from build123d import *

# Parameters (mm, degrees)
F1_DEPTH    = 7
F2_DEPTH    = 8
F3_R        = 3.99999
F4_T1_DEPTH = 20.2030500331
F5_R        = 5
F6_R        = 2.5
F7_DEPTH    = 10
F6_R_2      = 3
F8_DEPTH    = 4.6
F9_R        = 1.7
F10_DEPTH   = 7.001


# Not quite as in the source:
# - a fillet or chamfer that OpenCascade refuses, or shapes differently, is made with other operations: its cross-section is extruded or revolved along the edge and cut away or added
# - a fillet or chamfer is up to 0.001 mm smaller than in the source, because OpenCascade refuses the exact size


with BuildPart() as f1:
    # F0 (on Top) → F1 (new body)
    with BuildSketch(Plane.XY):
        Polygon((-25, -4), (25, -4), (25, 4), (-19.7969499669, 4), (-25, 4), align=None)
    extrude(amount=F1_DEPTH)

    # F0 (on Top) → F2 (join)
    with BuildSketch(Plane.XY):
        Polygon((-15.1648762861, 40.705181399), (-25, 4), (-19.7969499669, 4), (-10.3103645166, 39.4044188907), align=None)
    extrude(amount=F2_DEPTH)

    # F3 (radius 4 in the source; OpenCascade refuses exactly that, so slightly less here)
    f3_edges = [f1.edges().sort_by_distance(p)[0] for p in [
        (25, 4, 3.5),
        (25, -4, 3.5),
        (-25, -4, 3.5),
        (-10.310365, 39.404419, 4),
    ]]
    fillet(f3_edges, radius=F3_R)

    # F4: fillet of radius 5 on 1 edges, made by hand

    # F4_s2 → F4_t1 (cut)
    with BuildSketch(Plane.YZ.offset(-32.5)):
        with BuildLine():
            ThreePointArc((4, 7), (5.4188611699, 7.7434164903), (7, 8))
            Line((7, 8), (4, 8))
            Line((4, 8), (4, 7))
        make_face()
    extrude(amount=F4_T1_DEPTH, mode=Mode.SUBTRACT)

    # F5
    f5_edges = [f1.edges().sort_by_distance(p)[0] for p in [
        (-22.398475, 4, 7),
    ]]
    fillet(f5_edges, radius=F5_R)

    # F6 (on face) → F7 (cut)
    with BuildSketch(Plane(origin=(-24.3253175473, 6.5179491924, 0), x_dir=(-0.2588190451, -0.9659258263, 0), z_dir=(-0.9659258263, 0.2588190451, 0))):
        with Locations((-27.3932271776, 4)):
            Circle(F6_R)
    extrude(amount=-F7_DEPTH, mode=Mode.SUBTRACT)

    # F6 (on face) → F8 (cut)
    with BuildSketch(Plane(origin=(-24.3253175473, 6.5179491924, 0), x_dir=(-0.2588190451, -0.9659258263, 0), z_dir=(-0.9659258263, 0.2588190451, 0))):
        with Locations((-8.3932271776, 4)):
            Circle(F6_R_2)
    extrude(amount=-F8_DEPTH, mode=Mode.SUBTRACT)

    # F9 (on face) → F10 (cut, through all)
    with BuildSketch(Plane.XY.offset(7)):
        with Locations((21, 0)):
            Circle(F9_R)
    extrude(amount=-F10_DEPTH, mode=Mode.SUBTRACT)


solid = f1.part
The listing builds one solid part. Answer for the finished solid, in the listing's coordinates (mm). A direction names the side the tool comes from. Give positions to 0.01 mm unless a question says otherwise; leave off trailing zeros. Loops run counter-clockwise (first coordinate to the right, second up) from the corner with the lowest first, then second, coordinate; pieces in that order, holes last. Notation, with made-up numbers: (-34.75, 32) - (-15.75, 32) arc R21 ccw to (-15.75, 59) - close; hole circle Ø2 at (-11, 43.25). An arc over 180 degrees is marked (long way). Use one line per item in the form item = value.
1. Which of the six approach directions +Z, -Z, +X, -X, +Y, -Y give full straight-line access (tool end or side, diameter ignored) to faces 1 (the face through (-17.699, 13.475, 4.042)), 2 (the face through (0, -4, 3)), 3 (the face through (1, 4, 3))?
Calculated:
face_1 = none
face_2 = +Z, -Z, +X, -X, -Y
face_3 = +Z, -Z, +X
2. Find the intervals of material crossed by line 1 along Y through (x, z) = (21, 5.25); line 2 along Z through (x, y) = (-4, 1); line 3 along Y through (x, z) = (6, 5), in increasing order. Write a range as [from, to].
Calculated:
line_1 = [-4, -1.7], [1.7, 4]
line_2 = [0, 7]
line_3 = [-4, 4]
3. The mould has two halves that part along Y. Classify faces 4 (the face through (-20.014, 22.61, 3.944)), 5 (the face through (-14.2, 34.75, 4.11)), 6 (the face through (0, 0, 7)): pulls with the +Y half, pulls with the -Y half, needs draft (parallel to the pull), parting line crosses it, or undercut.
Calculated:
face_4 = pulls with the +Y half
face_5 = undercut
face_6 = needs draft
4. Section A-A on z = 5.5 is taken. Count the separate pieces of the cut face and the enclosed holes in it, then the cut area to 3 significant figures.
Calculated:
separate_pieces = 2
enclosed_holes = 1
area = 521 mm^2
5. Given pin 1 Ø4 at (x, y) = (4.5, -1) entering from +Z; pin 2 Ø1.5 at (y, z) = (24.5, 5.5) entering from -X; pin 3 Ø1.5 at (x, z) = (18, 7) entering from +Y, each flat-ended and moving along its own axis, determine where each tip first touches the part or whether it passes through.
Calculated:
pin_1 = 7
pin_2 = -19.71
pin_3 = 4
6. Section D-D on y = 5.5 is taken. Give the vertices of the cut face in (x, z).
Calculated:
outline = (-24.6, 0) - (-19.4, 0) - (-19.4, 7.77) - (-24.6, 7.77) - close
7. Section C-C on x = 17.5 is taken. Give the vertices of the cut face in (y, z).
Calculated:
outline = (-4, 0) - (4, 0) - (4, 7) - (-4, 7) - close
